Solid Edge part; units mm, degrees
sketch "Sketch1" plane through (0, 0, 0) normal (0, 0, 1) x (1, 0, 0)
  line L0 (-10.25, 9) -> (-10.25, -9)
  line L1 (-10.25, -9) -> (10.25, -9)
  line L2 (10.25, -9) -> (10.25, 9)
  line L3 (10.25, 9) -> (-10.25, 9)
extrude "Protrusion1" add sketch "Sketch1" along normal blind 1.6
sketch "Sketch2" plane through (0, 0, 1.6) normal (0, 0, 1) x (1, 0, 0)
  circle A0 centre (-10.25, 0) radius 1.2493
extrude "Cutout1" cut sketch "Sketch2" against normal up to vertex (1.6 mm away)
sketch "Sketch3" plane through (0, 0, 1.6) normal (0, 0, 1) x (1, 0, 0)
  line L0 (9.738, 8.9066) -> (-9.738, 8.9066)
  line L1 (-9.738, 8.9066) -> (-9.738, 6.9066)
  line L2 (-9.738, 6.9066) -> (9.738, 6.9066)
  line L3 (9.738, 6.9066) -> (9.738, 8.9066)
  line L4 (9.738, -8.9066) -> (9.738, -6.9066)
  line L5 (9.738, -6.9066) -> (-9.738, -6.9066)
  line L6 (-9.738, -6.9066) -> (-9.738, -8.9066)
  line L7 (-9.738, -8.9066) -> (9.738, -8.9066)
extrude "ExtrudedProtrusion_2" add sketch "Sketch3" against normal blind 8
sketch "Sketch4" plane through (0, 0, 1.6) normal (0, 0, 1) x (1, 0, 0)
  line L0 (11.0007, 5.6262) -> (-2.3727, 5.6262)
  line L1 (-2.3727, 5.6262) -> (-2.3727, -5.6262)
  line L2 (-2.3727, -5.6262) -> (11.0007, -5.6262)
  line L3 (11.0007, -5.6262) -> (11.0007, 5.6262)
extrude "ExtrudedProtrusion_3" add sketch "Sketch4" along normal blind 2
sketch "Sketch5" plane through (0, 0, -4.4) normal (0, 0, 1) x (1, 0, 0)
  line L0 (15.3, -10.375) -> (15.3, 10.375)
  line L1 (15.3, 10.375) -> (-17.25, 10.375)
  line L2 (-17.25, 10.375) -> (-17.25, -10.375)
  line L3 (-17.25, -10.375) -> (15.3, -10.375)
extrude "ExtrudedProtrusion_4" add sketch "Sketch5" along normal blind 1.6
sketch "Sketch6" plane through (-0.975, 0, -2.8) normal (0, 0, 1) x (1, 0, 0)
  circle A0 centre (-12.275, 6.35) radius 1.5
  circle A1 centre (-12.275, -6.35) radius 1.5
  arc A2 (13.8632, -5.7211) -> (16.275, -5.2788) centre (15.225, -6.35) cw
  line L0 (16.275, -7.4212) -> (16.275, -5.2788)
  arc A3 (16.275, -7.4212) -> (13.8632, -5.7211) centre (15.225, -6.35) cw
  arc A4 (16.275, 5.2788) -> (16.275, 7.4212) centre (15.225, 6.35) cw
  line L1 (16.275, 5.2788) -> (16.275, 7.4212)
extrude "Cutout2" cut sketch "Sketch6" against normal up to vertex (1.6 mm away)
sketch "Sketch7" plane through (4.314, 0, 3.6) normal (0, 0, 1) x (0, -1, 0)
  line L0 (-4.875, 8.936) -> (6.125, 8.936)
  line L1 (6.125, 8.936) -> (6.125, 5.936)
  line L2 (6.125, 5.936) -> (-4.875, 5.936)
  line L3 (-4.875, 5.936) -> (-4.875, 8.936)
extrude "ExtrudedProtrusion_5" add sketch "Sketch7" against normal blind 1
properties material "Steel"
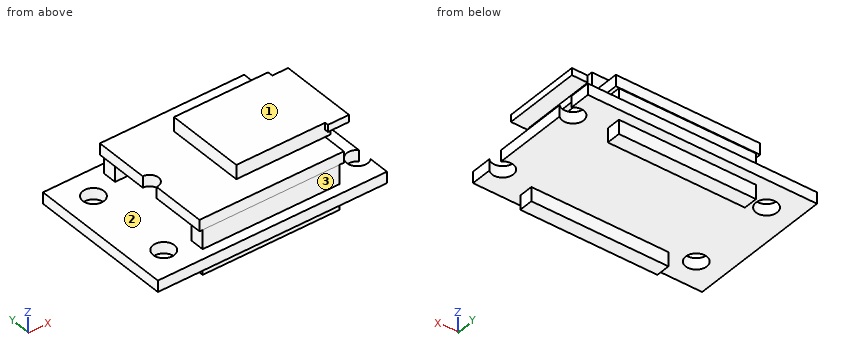
Source: CAD feature listing. Evaluate the final solid. Frame: model axes, mm. Face numbers are marked on the shaded views. Coordinates: 2 decimals unless noted, no trailing zeros. Order: outer loops, then holes, each group sorted by start corner. A loop starts at its lowest first (then second) coordinate and runs counter-clockwise, first axis right, second up. Notation, with made-up numbers: M 64,40.5 L 97,40.5 A22 ccw 97,69.5 Z; hole C 8,18.5 d11. An arc over 180 degrees is marked long. Write each question's results on one line, items separated by ' | '. Start each with the question number.
1. Section B-B, the plane x = 14.25. Return the cut outline in (y, z) (3 decimals).
2. Draft query along Z for the marked faces 1, 2 and 3. Return one class per face: +Z half, -Z half, draft (parallel to the pull), parting line (faces both ways), or undercut.
3. Section C-C, the plane z = -1.5. Return the cut outline in (x, y), then the cut area to 3 significant figures.
4. Pin query (flat end, axial travel): pin 1 (1.6 mm diameter, centred on y = 7.5, z = -5, fed in from +X); pin 2 (1 mm diameter, centred on y = 2, z = 2, fed in from +X); pin 3 (0.5 mm diameter, centred on y = 7, z = 0.5, fed in from -X); pin 4 (2 mm diameter, centred on x = -1, z = -5.5, fed in from -Y). Return the tip coordinate at first contact, or that it passes through.
5. Section A-A, the plane y = 6.35. Return the cut outline in (x, z), then the cut area to 3 significant figures.
6. Material intervals for L1, parallel to Y at x = 14.25, z = -3.4 (3 decimals); L2, parallel to Z at x = -1, y = 6; L3, parallel to Z at x = -2, y = -0.25, sorted ascending.
7. Section D-D, the plane y = 0. Return the cut outline in (x, z), then the cut area to 3 significant figures.
Solution:
1) outline: M -10.375,-4.4 L -7.85,-4.4 L -7.85,-2.8 L -10.375,-2.8 Z; M -4.85,-4.4 L 4.85,-4.4 L 4.85,-2.8 L -4.85,-2.8 Z; M 7.85,-4.4 L 10.375,-4.4 L 10.375,-2.8 L 7.85,-2.8 Z
2) face 1: +Z half | face 2: undercut | face 3: undercut
3) outline: M -9.74,-8.91 L 9.74,-8.91 L 9.74,-6.91 L -9.74,-6.91 Z; M -9.74,6.91 L 9.74,6.91 L 9.74,8.91 L -9.74,8.91 Z | area: 77.9 mm²
4) pin 1: x = 15.3 | pin 2: x = 11 | pin 3: x = -10.25 | pin 4: y = -8.91
5) outline: M -17.25,-4.4 L -14.75,-4.4 L -14.75,-2.8 L -17.25,-2.8 Z; M -11.75,-4.4 L 12.75,-4.4 L 12.75,-2.8 L -11.75,-2.8 Z; M -10.25,0 L 10.25,0 L 10.25,1.6 L -10.25,1.6 Z | area: 76.0 mm²
6) L1: -10.375 to -7.85, -4.85 to 4.85, 7.85 to 10.375 | L2: -4.4 to -2.8, 0 to 1.6 | L3: -4.4 to -2.8, 0 to 3.6
7) outline: M -17.25,-4.4 L 15.3,-4.4 L 15.3,-2.8 L -17.25,-2.8 Z; M -9,0 L 10.25,0 L 10.25,1.6 L 11,1.6 L 11,2.6 L 13.25,2.6 L 13.25,3.6 L -2.37,3.6 L -2.37,1.6 L -9,1.6 Z | area: 112 mm²
